Design review of the part built by this model. Coordinates are the model's own, in mm. A direction names the side the tool comes from. Coordinates: 2 decimals unless noted, no trailing zeros. Write each loop counter-clockwise with the first axis right and the second up, starting at its lowest first coordinate (ties: lowest second). Pieces come first, ordered by that corner, then holes. Notation, with made-up numbers: (41.5, 3) - (54.5, 3) arc R25 ccw to (54.5, 38) - close; hole circle Ø4 at (14, -28). An arc over 180 degrees is marked (long way). One line per item, written item: value.
from build123d import *

# Parameters (mm, degrees)
F0_W      = 152.4
F0_H      = 95.3626578227
F1_DEPTH  = 228.6
F2_T      = -2.54
F3_R      = 5.08
F4_R      = 35.2372499074
F5_DEPTH  = 25.4
F6_R      = 18.618406975
F6_R_2    = 16.5748786225
F6_R_3    = 8.7435651561
F6_R_4    = 17.3413047292
F7_DEPTH  = 25.4
F8_R      = 5.1423481667
F8_R_2    = 14.090646871
F8_R_3    = 6.6197884321
F8_R_4    = 15.148279019
F9_DEPTH  = 25.4
F10_W     = 119.2719545215
F10_H     = 14.1333565116
F11_DEPTH = 25.4
F12_W     = 94.5496149361
F12_H     = 14.0616036952
F13_DEPTH = 25.4
F14_W     = 102.1888470277
F14_H     = 7.4939653277
F15_DEPTH = 25.4


with BuildPart() as f1:
    # F0 (on Front) → F1 (new body)
    with BuildSketch(Plane.XZ):
        with Locations((-41.1360282451, 14.7424824536)):
            Rectangle(F0_W, F0_H)
    extrude(amount=F1_DEPTH)

    # F2
    f2_openings = [f1.faces().sort_by_distance(p)[0] for p in [
        (-41.136028, -114.3, -32.938846),
    ]]
    offset(amount=F2_T, openings=f2_openings)

    # F3
    f3_edges = [f1.edges().sort_by_distance(p)[0] for p in [
        (-114.796028, -114.3, 59.883811),
        (-114.796028, -226.06, 13.472482),
        (-41.136028, -226.06, 59.883811),
        (32.523972, -226.06, 13.472482),
        (-41.136028, -2.54, 59.883811),
        (-114.796028, -2.54, 13.472482),
        (35.063972, 0, 14.742482),
        (-117.336028, 0, 14.742482),
        (-117.336028, -228.6, 14.742482),
        (35.063972, -228.6, 14.742482),
        (32.523972, -2.54, 13.472482),
        (35.063972, -114.3, 62.423811),
        (-41.136028, -228.6, 62.423811),
        (-117.336028, -114.3, 62.423811),
        (32.523972, -114.3, 59.883811),
    ]]
    fillet(f3_edges, radius=F3_R)

    # F4 (on face) → F5 (cut)
    with BuildSketch(Plane.XY.offset(62.423811365)):
        with Locations((-13.0968187004, -43.1509837508)):
            Circle(F4_R)
    extrude(amount=-F5_DEPTH, mode=Mode.SUBTRACT)

    # F6 (on face) → F7 (cut)
    with BuildSketch(Plane.XY.offset(62.423811365)):
        with BuildLine():
            ThreePointArc((-112.2560282451, -52.3542664582), (-72.1481054557, -56.8578320674), (-50.6796549672, -22.681331262))
            ThreePointArc((-50.6796549672, -22.681331262), (-52.6104743381, -10.7325381795), (-58.2063964066, 0))
            Line((-58.2063964066, 0), (-112.2560282451, 0))
            Line((-112.2560282451, 0), (-112.2560282451, -52.3542664582))
        make_face()
        with Locations((-64.2905011773, -95.9484130144)):
            Circle(F6_R)
        with Locations((-3.6475341767, -153.4599065781)):
            Circle(F6_R_2)
        with Locations((-4.9036405981, -123.4000101686)):
            Circle(F6_R_3)
        with Locations((-56.035131216, -179.3635040522)):
            Circle(F6_R_4)
    extrude(amount=-F7_DEPTH, mode=Mode.SUBTRACT)

    # F8 (on face) → F9 (cut)
    with BuildSketch(Plane.XY.offset(62.423811365)):
        with Locations((-79.7442123294, -124.662168324)):
            Circle(F8_R)
        with Locations((-38.8632304966, -134.5197707415)):
            Circle(F8_R_2)
        with Locations((-88.7798666954, -159.4061106443)):
            Circle(F8_R_3)
        with Locations((-5.8542490005, -203.3631652594)):
            Circle(F8_R_4)
    extrude(amount=-F9_DEPTH, mode=Mode.SUBTRACT)

    # F10 (on face) → F11 (cut)
    with BuildSketch(Plane.XZ.offset(228.6)):
        with Locations((-38.4055124596, 46.7209592462)):
            Rectangle(F10_W, F10_H)
    extrude(amount=-F11_DEPTH, mode=Mode.SUBTRACT)

    # F12 (on face) → F13 (cut)
    with BuildSketch(Plane(origin=(-117.3360282451, 0, 0), x_dir=(0, -1, 0), z_dir=(-1, 0, 0))):
        with Locations((57.7809717506, 47.705097124)):
            Rectangle(F12_W, F12_H)
    extrude(amount=-F13_DEPTH, mode=Mode.SUBTRACT)

    # F14 (on face) → F15 (cut)
    with BuildSketch(Plane.YZ.offset(35.0639717549)):
        with Locations((-60.0578528829, 49.7737638652)):
            Rectangle(F14_W, F14_H)
    extrude(amount=-F15_DEPTH, mode=Mode.SUBTRACT)


solid = f1.part
1. Consider section B-B, the plane y = -208.5. Write out the cut boundary in (x, z).
Answer block:
outline: (-117.34, -32.94) - (-114.8, -32.94) - (-114.8, 54.8) arc R5.08 cw to (-109.72, 59.88) - (-20.1, 59.88) - (-20.1, 62.42) - (-112.26, 62.42) arc R5.08 ccw to (-117.34, 57.34) - close; (8.4, 59.88) - (27.44, 59.88) arc R5.08 cw to (32.52, 54.8) - (32.52, -32.94) - (35.06, -32.94) - (35.06, 57.34) arc R5.08 ccw to (29.98, 62.42) - (8.4, 62.42) - close
2. Insertion check: pin 1 Ø1.3 at (x, z) = (33, 51) entering from -Y; pin 2 Ø2 at (x, z) = (-116.5, 49) entering from +Y; pin 3 Ø4 at (x, y) = (-85.5, -133.5) entering from -Z; pin 4 Ø7.5 at (y, z) = (-37.5, 47.5) entering from +X. Each pin has a flat end and moves straight along its axis. Give the tip position at first contact, or say it passes through.
Answer block:
pin 1: stops at y = -228.02
pin 2: stops at y = -1.17
pin 3: stops at z = 59.88
pin 4: stops at x = 35.06
3. Consider section A-A, the plane z = 18. Write out the cut boundary in (x, y).
Answer block:
outline: (-117.34, -223.52) arc R5.08 ccw to (-112.26, -228.6) - (29.98, -228.6) arc R5.08 ccw to (35.06, -223.52) - (35.06, -5.08) arc R5.08 ccw to (29.98, 0) - (-112.26, 0) arc R5.08 ccw to (-117.34, -5.08) - close; hole (-114.8, -220.98) arc R5.08 ccw to (-109.72, -226.06) - (27.44, -226.06) arc R5.08 ccw to (32.52, -220.98) - (32.52, -7.62) arc R5.08 ccw to (27.44, -2.54) - (-109.72, -2.54) arc R5.08 ccw to (-114.8, -7.62) - close
4. Wall thickness on line 1 along Y through (x, z) = (27, 50); line 2 along X through (y, z) = (-161.5, -1); line 3 along Z through (x, y) = (-52, -200): over which ranges is each line inside the solid? List them lowest first.
Answer block:
line 1: y = -228.6 to -226.06, -2.54 to 0
line 2: x = -117.34 to -114.8, 32.52 to 35.06
line 3: z = 59.88 to 62.42
5. For faces 1 (the face through (-113.35, -4.07, 11.55)), 2 (the face through (-39.07, -19.34, 61.17)), list the 3-axis set-ups (+Z, -Z, +X, -X, +Y, -Y) from which the entire face can be reached by the end or side of a thin tool; tool diameter is ignored.
Answer block:
face 1: -Z
face 2: +Z, -Z
6. Consider section C-C, the plane y = -72. Write out the cut boundary in (x, z).
Answer block:
outline: (-117.34, -32.94) - (-114.8, -32.94) - (-114.8, 40.67) - (-117.34, 40.67) - close; (-117.34, 54.74) - (-114.8, 54.74) - (-114.8, 54.8) arc R5.08 cw to (-109.72, 59.88) - (-33.33, 59.88) - (-33.33, 62.42) - (-112.26, 62.42) arc R5.08 ccw to (-117.34, 57.34) - close; (7.14, 59.88) - (27.44, 59.88) arc R5.08 cw to (32.52, 54.8) - (32.52, 53.52) - (35.06, 53.52) - (35.06, 57.34) arc R5.08 ccw to (29.98, 62.42) - (7.14, 62.42) - close; (32.52, -32.94) - (35.06, -32.94) - (35.06, 46.03) - (32.52, 46.03) - close
7. Mouldability with a two-part tool opening along X and no side actions: class faces 3 (the face through (-115.887, -113.325, 60.896)), 4 (the face through (-42, -228.6, 3)), 5 (the face through (-82.665, -161.942, 61.172)) as released by +X, released by -X, zero draft, split by the parting line, or undercut.
Answer block:
face 3: released by -X
face 4: zero draft
face 5: undercut
